Work out the finished part from the listing and answer in its coordinate system (mm). Coordinates: 2 decimals unless noted, no trailing zeros. Order: outer loops, then holes, each group sorted by start corner. A loop starts at its lowest first (then second) coordinate and runs counter-clockwise, first axis right, second up. Notation, with made-up numbers: M 68.25,59.5 L 86.25,59.5 A34 cw 86.25,95.5 Z; hole C -37.5,81 d10. An arc over 180 degrees is marked long. Use a Markdown table: item, result.
from build123d import *

# Parameters (mm, degrees)
SKETCH1_R             = 25
SKETCH1_R_2           = 21
BOSS_EXTRUDE1_DEPTH   = 3.175
SKETCH1_R_3           = 2.5
SKETCH1_R_4           = 1.5
BOSS_EXTRUDE1_2_DEPTH = 3.175
BOSS_EXTRUDE2_DEPTH   = 3.175
CIRPATTERN1_COUNT     = 5
FILLET1_R             = 2
FILLET2_R             = 2


with BuildPart() as part:
    # Sketch1 → Boss-Extrude1 (new body)
    with BuildSketch(Plane.XY):
        Circle(SKETCH1_R)
        Circle(SKETCH1_R_2, mode=Mode.SUBTRACT)
    extrude(amount=BOSS_EXTRUDE1_DEPTH)



with BuildPart() as body_2:
    # Sketch1 → Boss-Extrude1 2 (new body)
    with BuildSketch(Plane.XY):
        Circle(SKETCH1_R_3)
        Circle(SKETCH1_R_4, mode=Mode.SUBTRACT)
    extrude(amount=BOSS_EXTRUDE1_2_DEPTH)


with BuildPart() as part_1:
    add(part.part)

    add(body_2.part)  # Boss-Extrude2 merges body 2
    # Sketch2 → Boss-Extrude2 (add)
    with BuildSketch(Plane.XY):
        with BuildLine():
            ThreePointArc((-1.5, 2), (-0.790569415, 2.371708245), (0, 2.5))
            Line((0, 2.5), (0, 21))
            ThreePointArc((0, 21), (-1.00113831, 20.976122666), (-2, 20.90454496))
            Line((-2, 20.90454496), (-1.5, 2))
        make_face()
        with BuildLine():
            Line((0, 21), (0, 2.5))
            ThreePointArc((0, 2.5), (0.790569415, 2.371708245), (1.5, 2))
            Line((1.5, 2), (2, 20.90454496))
            ThreePointArc((2, 20.90454496), (1.00113831, 20.976122666), (0, 21))
        make_face()
    boss_extrude2 = extrude(amount=BOSS_EXTRUDE2_DEPTH)

    # CirPattern1: Boss-Extrude2 ×5 about axis
    cirpattern1_axis = Axis((0, 0, 0), (0, 0, 1))
    for i in range(1, CIRPATTERN1_COUNT):
        add(boss_extrude2.rotate(cirpattern1_axis, i * 360 / CIRPATTERN1_COUNT))

    # Fillet1
    fillet1_edges = [part_1.edges().sort_by_distance(p)[0] for p in [
        (1.501772388, 2.067012363, 1.5875),
        (-1.501772388, 2.067012363, 1.5875),
        (-2.429918767, -0.789528467, 1.5875),
        (0, -2.554967791, 1.5875),
        (2.429918767, -0.789528467, 1.5875),
    ]]
    fillet(fillet1_edges, radius=FILLET1_R)

    # Fillet2
    fillet2_edges = [part_1.edges().sort_by_distance(p)[0] for p in [
        (-2, 20.90454496, 1.5875),
        (2, 20.90454496, 1.5875),
        (19.263369716, 8.361972685, 1.5875),
        (-20.499437693, 4.55774662, 1.5875),
        (-19.263369716, 8.361972685, 1.5875),
        (-10.669349245, -18.087702637, 1.5875),
        (-13.905417222, -15.736561628, 1.5875),
        (13.905417222, -15.736561628, 1.5875),
        (10.669349245, -18.087702637, 1.5875),
        (20.499437693, 4.55774662, 1.5875),
    ]]
    fillet(fillet2_edges, radius=FILLET2_R)


solid = part_1.part
(1) A cutting plane is placed at D-D (x = -22). Determine the outline of the cut face in (y, z) (3 decimals), then the cut area to 3 significant figures.
Conclusion:
| item | result |
|---|---|
| outline | M -11.874,0 L 11.874,0 L 11.874,3.175 L -11.874,3.175 Z |
| area | 75.4 mm2 |
(2) Given P1, Ø5, axis at x = 0, y = 0, coming from the +Z side (3 decimals); P2, Ø1, axis at y = -2.5, z = 1.5, coming from the -X side; P3, Ø1, axis at x = 16.5, y = -11.5, coming from the +Z side, each flat-ended and moving along its own axis, determine where each tip first touches the part or whether it passes through.
Conclusion:
| item | result |
|---|---|
| P1 | z = 3.175 |
| P2 | x = -24.92 |
| P3 | through |
(3) A cutting plane is placed at B-B (x = 0). Determine the outline of the cut face in (y, z) (3 decimals).
Conclusion:
| item | result |
|---|---|
| outline | M -25,0 L -21,0 L -21,3.175 L -25,3.175 Z; M -4.087,0 L -1.5,0 L -1.5,3.175 L -4.087,3.175 Z; M 1.5,0 L 25,0 L 25,3.175 L 1.5,3.175 Z |
(4) A cutting plane is placed at A-A (z = 1.85). Give the number of separate pieces and of enclosed holes in the cut face, then the cut area to 3 significant figures.
Conclusion:
| item | result |
|---|---|
| separate pieces | 1 |
| enclosed holes | 6 |
| area | 939 mm2 |
(5) Determine the mould class of faces 1 (the cylindrical face through (23.846, 7.509, 1.565)), 2 (the flat face through (-4, -3.3, 3.175)), 3 (the flat face through (-11.866, 2.003, 1.565)) for opening direction Y: pulls with the +Y half, pulls with the -Y half, needs draft (parallel to the pull), parting line crosses it, or undercut.
Conclusion:
| item | result |
|---|---|
| face 1 | parting line crosses it |
| face 2 | needs draft |
| face 3 | undercut |
(6) A cutting plane is placed at C-C (y = -11). Determine the outline of the cut face in (x, z) (3 decimals), then the cut area to 3 significant figures.
Conclusion:
| item | result |
|---|---|
| outline | M -22.45,0 L -17.889,0 L -17.889,3.175 L -22.45,3.175 Z; M -10.269,0 L -5.801,0 L -5.801,3.175 L -10.269,3.175 Z; M 5.801,0 L 10.269,0 L 10.269,3.175 L 5.801,3.175 Z; M 17.889,0 L 22.45,0 L 22.45,3.175 L 17.889,3.175 Z |
| area | 57.3 mm2 |
(7) Straight lines are drawn through the part: L1, parallel to Y at x = 0, z = 1.8; L2, parallel to Y at x = 10, z = 1.85; L3, parallel to X at y = 16.5, z = 1.55. For each, find the intervals that lie inside material, in ascending order.
Conclusion:
| item | result |
|---|---|
| L1 | -25 to -21, -4.09 to -1.5, 1.5 to 25 |
| L2 | -22.91 to -10.65, 1.45 to 5.08, 18.47 to 22.91 |
| L3 | -18.78 to -12.99, -1.88 to 1.88, 12.99 to 18.78 |
